Can you work these out from the model? Positions are in its coordinate system, mm. Face numbers are marked on the shaded views. Give positions to 0.01 mm unless a question says otherwise; leave off trailing zeros. Loops run counter-clockwise (first coordinate to the right, second up) from the corner with the lowest first, then second, coordinate; pieces in that order, holes last. Notation, with made-up numbers: (46.5, 7) - (50.5, 7) arc R28 ccw to (50.5, 38) - close; hole circle Ø7 at (66, -7). An arc over 180 degrees is marked (long way). Answer in a Markdown table with one row per item.
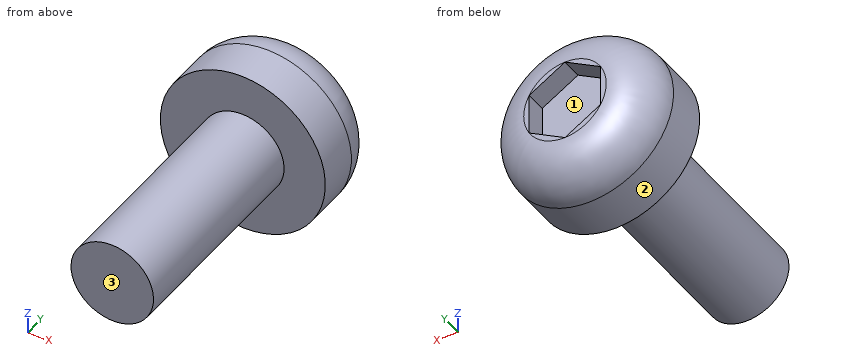
from build123d import *

# Parameters (mm, degrees)
SKETCH1_R           = 1
BOSS_EXTRUDE1_DEPTH = 5
SKETCH2_R           = 2
BOSS_EXTRUDE2_DEPTH = 2
FILLET1_R           = 1
CUT_EXTRUDE1_DEPTH  = 0.5


with BuildPart() as part:
    # Sketch1 → Boss-Extrude1 (new body)
    with BuildSketch(Plane(origin=(0, 0, 0), x_dir=(1, 0, 0), z_dir=(0, 1, 0))):
        with Locations(Location((0, 0, 0), (0, 0, 270))):
            Circle(SKETCH1_R)
    extrude(amount=BOSS_EXTRUDE1_DEPTH)

    # Sketch2 → Boss-Extrude2 (add)
    with BuildSketch(Plane(origin=(0, 5, 0), x_dir=(1, 0, 0), z_dir=(0, 1, 0))):
        with Locations(Location((0, 0, 0), (0, 0, 270))):
            Circle(SKETCH2_R)
    extrude(amount=BOSS_EXTRUDE2_DEPTH)

    # Fillet1
    fillet1_edges = [part.edges().sort_by_distance(p)[0] for p in [
        (0, 7, -2),
    ]]
    fillet(fillet1_edges, radius=FILLET1_R)

    # Sketch3 → Cut-Extrude1 (cut)
    with BuildSketch(Plane(origin=(0, 7, 0), x_dir=(1, 0, 0), z_dir=(0, 1, 0))):
        Polygon((-0.866025404, 0.5), (0, 0), (0, 1), align=None)
        Polygon((-0.866025404, -0.5), (0, 0), (-0.866025404, 0.5), align=None)
        Polygon((-0.866025404, -0.5), (0, -1), (0, 0), align=None)
        Polygon((0, 0), (0, -1), (0.866025404, -0.5), align=None)
        Polygon((0.866025404, 0.5), (0, 0), (0.866025404, -0.5), align=None)
        Polygon((0, 1), (0, 0), (0.866025404, 0.5), align=None)
    extrude(amount=-CUT_EXTRUDE1_DEPTH, mode=Mode.SUBTRACT)


solid = part.part
Q1. If we mould it in two halves opening along X, with no side actions, what happens to the marked faces 1, 2 and 3? For each: released by +X, released by -X, zero draft, split by the parting line, or undercut.
Checked values:
| item | result |
|---|---|
| face 1 | undercut |
| face 2 | split by the parting line |
| face 3 | zero draft |
Q2. If I drill on line 1 (X direction, y = 5.25, z = -0.1); line 2 (Y direction, x = -0.05, z = 1.2); line 3 (X direction, y = 6.5, z = 1.6), over which ranges is the centre line in solid material (lowest first)? Write a range as [from, to].
Checked values:
| item | result |
|---|---|
| line 1 | x = [-2, 2] |
| line 2 | y = [5, 6.98] |
| line 3 | x = [-0.96, 0.96] |
Q3. For pin 1 (1 mm diameter, centred on x = 0, y = 1.5, fed in from -Z); pin 2 (0.6 mm diameter, centred on y = 7, z = 0, fed in from +X); pin 3 (2 mm diameter, centred on y = 1, z = 1, fed in from +X), each with a flat end and sliding along its axis, tell me the tip position at first contact or that it passes through.
Checked values:
| item | result |
|---|---|
| pin 1 | stops at z = -1 |
| pin 2 | stops at x = 1.71 |
| pin 3 | stops at x = 1 |
Q4. Imagine slicing it at A-A, the plane y = 3. Write out the boundary of the cut face in (x, z).
Checked values:
| item | result |
|---|---|
| outline | circle Ø2 at (0, 0) |
